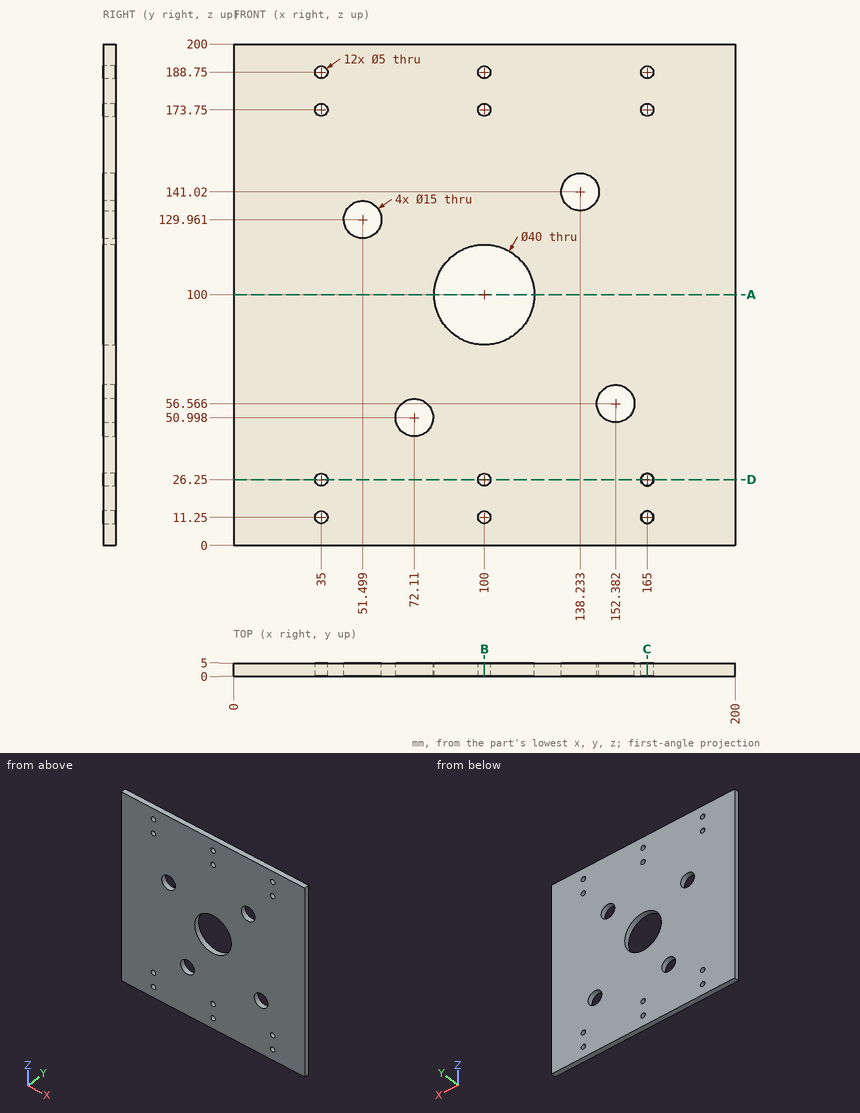
Could you check a few things on this drawing? It's one solid part, dimensions in mm from its lowest x, y, z. Round coordinates to 2 decimals unless told otherwise and drop trailing zeros. Order: outer loops, then holes, each group sorted by start corner. A loop starts at its lowest first (then second) coordinate and runs counter-clockwise, first axis right, second up.
(1) Imagine slicing it at C-C (x = 165). Write out the boundary of the cut face in (y, z).
Response values:
outline: (0, 0) - (5, 0) - (5, 8.75) - (0, 8.75) - close; (0, 13.75) - (5, 13.75) - (5, 23.75) - (0, 23.75) - close; (0, 28.75) - (5, 28.75) - (5, 171.25) - (0, 171.25) - close; (0, 176.25) - (5, 176.25) - (5, 186.25) - (0, 186.25) - close; (0, 191.25) - (5, 191.25) - (5, 200) - (0, 200) - close
(2) Imagine slicing it at A-A (z = 100). Write out the boundary of the cut face in (x, y), plus the area to 3 significant figures.
Response values:
outline: (0, 0) - (80, 0) - (80, 5) - (0, 5) - close; (120, 0) - (200, 0) - (200, 5) - (120, 5) - close
area: 800 mm2
(3) Imagine slicing it at B-B (x = 100). Write out the boundary of the cut face in (y, z).
Response values:
outline: (0, 0) - (5, 0) - (5, 8.75) - (0, 8.75) - close; (0, 13.75) - (5, 13.75) - (5, 23.75) - (0, 23.75) - close; (0, 28.75) - (5, 28.75) - (5, 80) - (0, 80) - close; (0, 120) - (5, 120) - (5, 171.25) - (0, 171.25) - close; (0, 176.25) - (5, 176.25) - (5, 186.25) - (0, 186.25) - close; (0, 191.25) - (5, 191.25) - (5, 200) - (0, 200) - close
(4) Imagine slicing it at D-D (z = 26.25). Write out the boundary of the cut face in (x, y).
Response values:
outline: (0, 0) - (32.5, 0) - (32.5, 5) - (0, 5) - close; (37.5, 0) - (97.5, 0) - (97.5, 5) - (37.5, 5) - close; (102.5, 0) - (162.5, 0) - (162.5, 5) - (102.5, 5) - close; (167.5, 0) - (200, 0) - (200, 5) - (167.5, 5) - close
(5) I'm going to push a flat-ended pin straight in: pin 1 (4 mm diameter, centred on x = 100, z = 26.25, fed in from -Y). Where does the tip first touch, or does it pass through?
Response values:
pin 1: passes through
(6) Please list where these lines run through material, in increasing order: line 1 along X through (y, z) = (3, 26.25); line 2 along Z through (x, y) = (165, 2.9); line 3 along X through (y, z) = (4.2, 101) (1 decimal).
Response values:
line 1: x = 0 to 32.5, 37.5 to 97.5, 102.5 to 162.5, 167.5 to 200
line 2: z = 0 to 8.75, 13.75 to 23.75, 28.75 to 171.25, 176.25 to 186.25, 191.25 to 200
line 3: x = 0 to 80, 120 to 200
